Autodesk Inventor part; units mm, degrees
ref_plane "Arbeitsebene1" through (0, 0, 0) normal (0, 0, -1) x (-1, 0, 0)
ref_plane "YZ Plane" through (0, 0, 0) normal (1, 0, 0) x (0, 1, 0)
ref_plane "XZ Plane" through (0, 0, 0) normal (0, 1, 0) x (-1, 0, 0)
ref_plane "Arbeitsebene1" through (0, 0, 0) normal (0, 0, -1) x (-1, 0, 0)
sketch "Skizze5" plane through (0, 0, 0) normal (0, 0, -1) x (-1, 0, 0)
  line L0 (29.5, 13.05) -> (-29.5, 13.05)
  line L1 (-29.5, 13.05) -> (-29.5, -13.05)
  line L2 (-29.5, -13.05) -> (29.5, -13.05)
  line L3 (29.5, -13.05) -> (29.5, 13.05)
  point P0 (0, 0)
  point P1 (29.5, 0)
  point P2 (0, -13.05)
  dimension "d70" = 26.1
  dimension "d71" = 59
extrude "Extrusion5" add sketch "Skizze5" along normal blind 1
sketch "Skizze4" plane through (0, 0, 0) normal (0, 0, -1) x (-1, 0, 0)
  line L0 (22.9, 13.05) -> (-17.8, 13.05)
  line L1 (-17.8, 13.05) -> (-17.8, 10.55)
  line L2 (-17.8, 10.55) -> (22.9, 10.55)
  line L3 (22.9, 10.55) -> (22.9, 13.05)
  line L4 (29.5, -13.05) -> (29.5, 13.05)
  line L5 (-29.5, -13.05) -> (29.5, -13.05)
  line L6 (29.5, 13.05) -> (-29.5, 13.05)
  line L7 (22.9, -13.05) -> (-27.6, -13.05)
  line L8 (-27.6, -13.05) -> (-27.6, -10.55)
  line L9 (-27.6, -10.55) -> (22.9, -10.55)
  line L10 (22.9, -10.55) -> (22.9, -13.05)
  dimension "d68" = 40.7
  dimension "d69" = 2.5
  dimension "d77" = 6.6
  dimension "d78" = 50.5
extrude "Extrusion4" add sketch "Skizze4" against normal blind 2.5
sketch "Skizze6" plane through (0, 0, -1) normal (0, 0, -1) x (-1, 0, 0)
  line L0 (22.2, -9) -> (4.2, -9)
  line L1 (4.2, -9) -> (4.2, 9)
  line L2 (4.2, 9) -> (22.2, 9)
  line L3 (22.2, 9) -> (22.2, -9)
  line L4 (29.5, -13.05) -> (29.5, 13.05)
  point P0 (0, 0)
  point P1 (4.2, 0)
  dimension "d26" = 18
  dimension "d27" = 18
  dimension "d72" = 7.3
extrude "Extrusion6" add sketch "Skizze6" along normal blind 3.2
sketch "Skizze7" plane through (0, 0, -1) normal (0, 0, -1) x (-1, 0, 0)
  line L0 (-24.3, -6.05) -> (-29.5, -6.05)
  line L1 (-29.5, -6.05) -> (-29.5, 1.45)
  line L2 (-29.5, 1.45) -> (-24.3, 1.45)
  line L3 (-24.3, 1.45) -> (-24.3, -6.05)
  line L4 (-29.5, 13.05) -> (-29.5, -13.05)
  line L5 (-29.5, -13.05) -> (29.5, -13.05)
  point P0 (0, 0)
  dimension "d31" = 7.5
  dimension "d32" = 5.2
  dimension "d73" = 7
  dimension "d74" = 0
extrude "Extrusion7" add sketch "Skizze7" along normal blind 2.6
sketch "Skizze8" plane through (0, 0, -1) normal (0, 0, -1) x (-1, 0, 0)
  line L0 (-19.5, 5.45) -> (-27.5, 5.45)
  line L1 (-27.5, 5.45) -> (-27.5, 13.05)
  line L2 (-27.5, 13.05) -> (-19.5, 13.05)
  line L3 (-19.5, 13.05) -> (-19.5, 5.45)
  line L4 (29.5, 13.05) -> (-29.5, 13.05)
  line L5 (-29.5, 13.05) -> (-29.5, 1.45)
  point P0 (0, 0)
  dimension "d36" = 7.6
  dimension "d37" = 8
  dimension "d75" = 0
  dimension "d79" = 2
extrude "Extrusion8" add sketch "Skizze8" along normal blind 5.6
properties part number "Dummy_ESP32_LOLIN_D32"
CAD build for the part. Positions are in the model's coordinates, mm. A direction names the side the tool comes from. Round coordinates to 2 decimals unless told otherwise and drop trailing zeros. Write each loop counter-clockwise with the first axis right and the second up, starting at its lowest first coordinate (ties: lowest second). Pieces come first, ordered by that corner, then holes. Notation, with made-up numbers: (35.25, 71.5) - (48.25, 71.5) arc R19 cw to (48.25, 92.5) - close; hole circle Ø8 at (-11.75, 10). An arc over 180 degrees is marked (long way). Return JSON: item names as keys, results as strings. Group by question number.
Item 1: Flat gauge pins, fed straight in: pin 1 Ø2 at (x, z) = (27, -2.5) entering from -Y; pin 2 Ø1.2 at (y, z) = (-12, 1.5) entering from -X; pin 3 Ø2.5 at (x, z) = (-10.5, -2.5) entering from +Y; pin 4 Ø1.5 at (y, z) = (-8, 1) entering from +X. Where does each tip first touch, or does it go through?
Item 2: Band-saw the part on A-A on x = -18. List the corners of the cut face in (y, z).
Item 3: Probe probe 1 along Y at (x, z) = (10.5, 1.75); probe 2 along Z at (x, y) = (-26, 12); probe 3 along X at (y, z) = (-6.5, -2.25). List the from-to ranges inside material, lowest first.
Item 4: Band-saw the part on C-C on z = -1.75. List the corners of the cut face in (x, y), plus the area to 3 significant figures.
Item 5: Mould opens along X. For faces 1 (the face through (29.5, 0, -1)), 2 (the face through (0, 0, -1)), 3 (the face through (3, -12, 2.5)), 4 (the face through (-22.9, -12, 1)) say: +X half, -X half, draft (parallel to the pull), parting line (faces both ways), or undercut.
Item 6: Band-saw the part on B-B on y = -1. List the corners of the cut face in (x, z), plus the area to 3 significant figures.
Item 7: Band-saw the part on D-D on x = 22.5. List the corners of the cut face in (y, z), plus the area to 3 significant figures.
Item 8: 3-axis set-ups, long thin cutter, end or side, ignore diameter. For faces 5 (the face through (27.5, 9, -4)), 6 (the face through (23, 5.45, -4)), 7 (the face through (3, -10.55, 1)), 8 (the face through (-22.2, 0, -3)): which of +Z, -Z, +X, -X, +Y, -Y reach the whole face in a straight line?
Resolved:
{
 "1": {"pin 1": "stops at y = -6.05", "pin 2": "stops at x = -22.9", "pin 3": "stops at y = 9", "pin 4": "passes through"},
 "2": {"outline": "(-13.05, -1) - (-9, -1) - (-9, -4.2) - (9, -4.2) - (9, -1) - (13.05, -1) - (13.05, 2.5) - (10.55, 2.5) - (10.55, 0) - (-10.55, 0) - (-10.55, 2.5) - (-13.05, 2.5) - close"},
 "3": {"probe 1": "y = -13.05 to -10.55, 10.55 to 13.05", "probe 2": "z = -1 to 0", "probe 3": "x = -22.2 to -4.2"},
 "4": {"outline": "(-22.2, -9) - (-4.2, -9) - (-4.2, 9) - (-22.2, 9) - close; (19.5, 5.45) - (27.5, 5.45) - (27.5, 13.05) - (19.5, 13.05) - close; (24.3, -6.05) - (29.5, -6.05) - (29.5, 1.45) - (24.3, 1.45) - close", "area": "424 mm²"},
 "5": {"face 1": "+X half", "face 2": "undercut", "face 3": "draft", "face 4": "-X half"},
 "6": {"outline": "(-29.5, -1) - (-22.2, -1) - (-22.2, -4.2) - (-4.2, -4.2) - (-4.2, -1) - (24.3, -1) - (24.3, -3.6) - (29.5, -3.6) - (29.5, 0) - (-29.5, 0) - close", "area": "130 mm²"},
 "7": {"outline": "(-13.05, -1) - (5.45, -1) - (5.45, -6.6) - (13.05, -6.6) - (13.05, 0) - (-10.55, 0) - (-10.55, 2.5) - (-13.05, 2.5) - close", "area": "74.9 mm²"},
 "8": {"face 5": "-Z, +X, +Y", "face 6": "-Z, +X", "face 7": "+Z, +X, -X", "face 8": "-Z, -X, +Y, -Y"}
}
